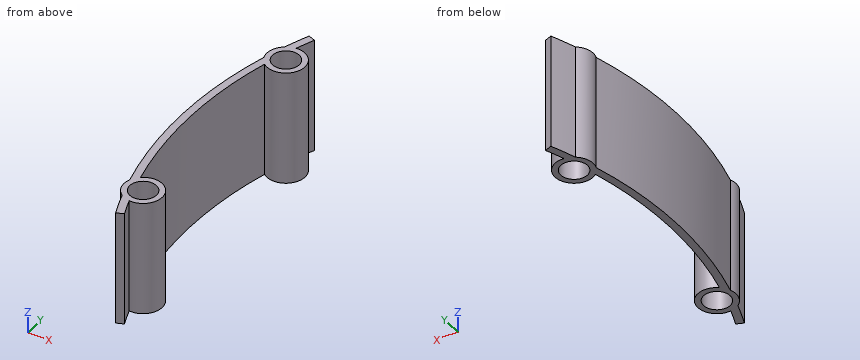
from build123d import *

# Parameters (mm, degrees)
SKETCH1_R           = 3.5
BOSS_EXTRUDE1_DEPTH = 30


with BuildPart() as part:
    # Sketch1 → Boss-Extrude1 (new body)
    with BuildSketch(Plane.XY):
        with BuildLine():
            Line((7.757871849, 40), (9.612864898, 39.252336449))
            ThreePointArc((9.612864898, 39.252336449), (8.688014127, 36.874834695), (7.821195192, 34.475566375))
            ThreePointArc((7.821195192, 34.475566375), (13.105433831, 28.067961165), (5.171505388, 25.611670876))
            ThreePointArc((5.171505388, 25.611670876), (2, 0), (5.171505388, -25.611670876))
            ThreePointArc((5.171505388, -25.611670876), (13.105433831, -28.067961165), (7.821195192, -34.475566375))
            ThreePointArc((7.821195192, -34.475566375), (8.688014127, -36.874834695), (9.612864898, -39.252336449))
            Line((9.612864898, -39.252336449), (7.757871849, -40))
            ThreePointArc((7.757871849, -40), (6.527354129, -36.800100973), (5.399981488, -33.562423012))
            ThreePointArc((5.399981488, -33.562423012), (3.524355651, -30.932038835), (3.648663608, -27.703813202))
            ThreePointArc((3.648663608, -27.703813202), (0, 0), (3.648663608, 27.703813202))
            ThreePointArc((3.648663608, 27.703813202), (3.524355651, 30.932038835), (5.399981488, 33.562423012))
            ThreePointArc((5.399981488, 33.562423012), (6.527354129, 36.800100973), (7.757871849, 40))
        make_face()
        with Locations((8.314894741, 29.5)):
            Circle(SKETCH1_R, mode=Mode.SUBTRACT)
        with Locations((8.314894741, -29.5)):
            Circle(SKETCH1_R, mode=Mode.SUBTRACT)
    extrude(amount=BOSS_EXTRUDE1_DEPTH)


solid = part.part
The model under review builds one solid part; all positions refer to its coordinate system, in mm. Give positions to 0.01 mm unless a question says otherwise; leave off trailing zeros. Loops run counter-clockwise (first coordinate to the right, second up) from the corner with the lowest first, then second, coordinate; pieces in that order, holes last. Notation, with made-up numbers: (30.25, 51) -> (63.25, 51) arc R16 cw to (63.25, 82) -> close; hole circle Ø8 at (4, 31). An arc over 180 degrees is marked (long way). Answer as a JSON object with one key per item and string values. Group by question number.
Q1. Wall thickness on line 1 along X through (y, z) = (27.5, 3.25); line 2 along X through (y, z) = (-27, 4.75); line 3 along Y through (x, z) = (12, 4): over which ranges is each line inside the solid? List them lowest first.
Q2. Take a section at C-C (x = 7). Write out the cut boundary in (y, z).
Q3. Insertion check: pin 1 (5 mm diameter, centred on y = 23.5, z = 15, fed in from -X); pin 2 (6 mm diameter, centred on y = -27.5, z = 21, fed in from -X); pin 3 (1.5 mm diameter, centred on y = 7.5, z = 17.5, fed in from -X); pin 4 (4 mm diameter, centred on x = 8.31, y = 29.5, fed in from -Z). Each pin has a flat end and moves straight along its axis. Give the tip position at first contact, or say it passes through.
Q4. Take a section at A-A (y = -29.5). Write out the cut boundary in (x, z), plus the area to 3 significant figures.
Q5. Take a section at B-B (z = 12.5). Write out the cut boundary in (x, y).
Q6. Take a section at D-D (y = 28.5). Write out the cut boundary in (x, z).
Answer below:
{
 "1": {"line 1": "x = 3.59 to 5.44, 11.19 to 12.9", "line 2": "x = 3.46 to 5.87, 10.76 to 12.65", "line 3": "y = -32.88 to -26.12, 26.12 to 32.88"},
 "2": {"outline": "(-38.07, 0) -> (-32.74, 0) -> (-32.74, 30) -> (-38.07, 30) -> close; (-26.26, 0) -> (-24.68, 0) -> (-24.68, 30) -> (-26.26, 30) -> close; (24.68, 0) -> (26.26, 0) -> (26.26, 30) -> (24.68, 30) -> close; (32.74, 0) -> (38.07, 0) -> (38.07, 30) -> (32.74, 30) -> close"},
 "3": {"pin 1": "stops at x = 2.08", "pin 2": "stops at x = 2.84", "pin 3": "stops at x = 0.21", "pin 4": "passes through"},
 "4": {"outline": "(3.31, 0) -> (4.81, 0) -> (4.81, 30) -> (3.31, 30) -> close; (11.81, 0) -> (13.31, 0) -> (13.31, 30) -> (11.81, 30) -> close", "area": "90.0 mm2"},
 "5": {"outline": "(3.65, -27.7) arc R5 ccw to (5.4, -33.56) arc R107 ccw to (7.76, -40) -> (9.61, -39.25) arc R105 cw to (7.82, -34.48) arc R5 ccw (long way) to (5.17, -25.61) arc R105 cw to (5.17, 25.61) arc R5 ccw (long way) to (7.82, 34.48) arc R105 cw to (9.61, 39.25) -> (7.76, 40) arc R107 ccw to (5.4, 33.56) arc R5 ccw to (3.65, 27.7) arc R107 ccw to start; hole circle Ø7 at (8.31, -29.5); hole circle Ø7 at (8.31, 29.5)"},
 "6": {"outline": "(3.42, 0) -> (4.96, 0) -> (4.96, 30) -> (3.42, 30) -> close; (11.67, 0) -> (13.21, 0) -> (13.21, 30) -> (11.67, 30) -> close"}
}
